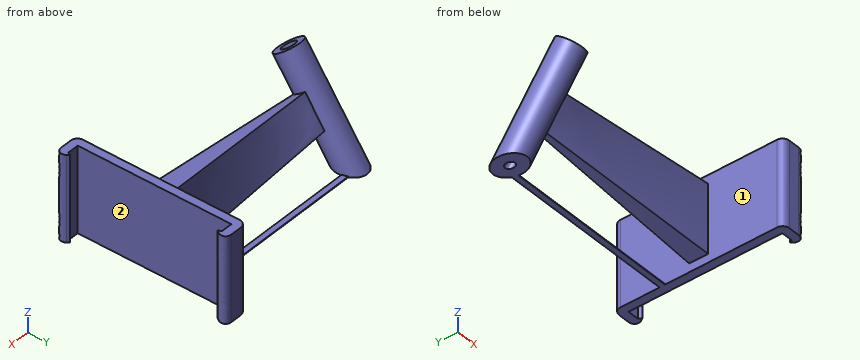
```python
from build123d import *

# Parameters (mm, degrees)
F1_DEPTH  = 25
F4_W      = 5.5
F4_H      = 20
F9_W      = 27.424
F9_H      = 9.749
F10_DEPTH = 25
F11_W     = 1.6
F11_H     = 0.2


with BuildPart() as f1:
    # F0 (on Top) → F1 (new body)
    with BuildSketch(Plane.XY):
        with BuildLine():
            Line((0, -22.4), (0, 0))
            Line((0, 0), (0, 22.4))
            Line((0, 22.4), (3.3, 22.4))
            Line((3.3, 22.4), (3.7377447908, 21.5009007295))
            Line((3.7377447908, 21.5009007295), (4.2500217799, 22.1906429157))
            add(Edge.make_bspline(
                [(4.2500217799, 22.1906429157), (4.5826178906, 22.638458401), (4.7916104177, 24.2520123151), (3.4845446819, 24.8), (2.8422182777, 24.8)],
                knots=[0, 0, 0, 0, 0.5032486408, 1, 1, 1, 1], degree=3))
            Line((2.8422182777, 24.8), (-0.4, 24.8))
            ThreePointArc((-0.4, 24.8), (-1.8142135624, 24.2142135624), (-2.4, 22.8))
            Line((-2.4, 22.8), (-2.4, 0))
            Line((-2.4, 0), (-2.4, -22.8))
            ThreePointArc((-2.4, -22.8), (-1.8142135624, -24.2142135624), (-0.4, -24.8))
            Line((-0.4, -24.8), (2.8422182777, -24.8))
            add(Edge.make_bspline(
                [(4.2500217799, -22.1906429157), (4.5826178906, -22.638458401), (4.7916104177, -24.2520123151), (3.4845446819, -24.8), (2.8422182777, -24.8)],
                knots=[0, 0, 0, 0, 0.5032486408, 1, 1, 1, 1], degree=3))
            Line((4.2500217799, -22.1906429157), (3.7377447908, -21.5009007295))
            Line((3.7377447908, -21.5009007295), (3.3, -22.4))
            Line((3.3, -22.4), (0, -22.4))
        make_face()
    extrude(amount=F1_DEPTH)

    # F4 (on face) → F5 section 0
    with BuildSketch(Plane(origin=(-2.4, 0, 0), x_dir=(0, -1, 0), z_dir=(-1, 0, 0))):
        with Locations((0, 12.5)):
            Rectangle(F4_W, F4_H)
    # F3 (on offset) → F5 section 1
    with BuildSketch(Plane.YZ.offset(-55)):
        Polygon((4.5061862703, 9.812834642), (-1.2295780932, 18.0043550849), (-4.5061862703, 15.7100493395), (1.2295780932, 7.5185288966), align=None)
    loft()

    # F7 (on face) → F8 (revolve)
    with BuildSketch(Plane(origin=(0, 5.9959164346, 4.198385886), x_dir=(1, 0, 0), z_dir=(0, -0.8191520443, -0.5735764364))):
        Polygon((-59.2, -9.0757438921), (-59.2, 15.9242561079), (-60.1, 15.9242561079), (-60.1, 25.9242561079), (-62.1, 25.9242561079), (-62.1, -9.0757438921), align=None)
    revolve(axis=Axis((-58, -0.1314634537, 12.94919126), (0, -0.5735764364, 0.8191520443)))

    # F9 (on Front) → F10 (cut)
    with BuildSketch(Plane.XZ):
        with Locations((-57.2514572268, -4.8745)):
            Rectangle(F9_W, F9_H)
    extrude(amount=-F10_DEPTH, mode=Mode.SUBTRACT)

    # F11 (on face) → F12 (join, up to the next surface of F1)
    with BuildSketch(Plane(origin=(-2.4, 0, 0), x_dir=(0, -1, 0), z_dir=(-1, 0, 0))):
        with Locations((-10.6029133692, 0.1)):
            Rectangle(F11_W, F11_H)
    extrude(until=Until.NEXT)


solid = f1.part
```
Part model, mm, in its own coordinate system. Face numbers are marked on the shaded views. Round coordinates to 2 decimals unless told otherwise and drop trailing zeros. Order: outer loops, then holes, each group sorted by start corner. A loop starts at its lowest first (then second) coordinate and runs counter-clockwise, first axis right, second up. Notation, with made-up numbers: M 19,41 L 31,41 A23 cw 31,71 Z; hole C 5,56.25 d9. An arc over 180 degrees is marked long. Put each result on its own line as item: value. Start each with the question number.
1. Slice it at A-A on z = 6.25. State how many separate pieces and enclosed holes the cut face has, then the cut area to 3 significant figures.
2. Drill centre lines: probe 1 along Z at (x, y) = (-33.5, 11); probe 2 along X at (y, z) = (12.5, 21.25); probe 3 along X at (y, z) = (22.5, 15). Where is each one in solid material? Low to high. Write a range as [from, to].
3. Drop flat-ended pins along their axis: pin 1 (2 mm diameter, centred on y = -11, z = 11, fed in from -X); pin 2 (4 mm diameter, centred on x = -49, y = 9, fed in from +Z); pin 3 (3.5 mm diameter, centred on x = 1.5, y = -5.5, fed in from +Z); pin 4 (6 mm diameter, centred on x = -36.5, y = -8, fed in from -Z). Give the stop position or say it passes through.
4. Slice it at B-B on y = 18. List the corners of the cut face in (x, z).
5. Two-plate mould, pull along Y, no slides. Class the marked faces 1 and 2: +Y half, -Y half, draft (parallel to the pull), parting line (faces both ways), or undercut.
Findings:
1. separate pieces: 2
1. enclosed holes: 1
1. area: 358 mm2
2. probe 1: [0, 0.2]
2. probe 2: [-2.4, 0]
2. probe 3: [-2.4, 4.42]
3. pin 1: x = -2.4
3. pin 2: z = 0.2
3. pin 3: z = 25
3. pin 4: through
4. outline: M -2.4,0 L 0,0 L 0,25 L -2.4,25 Z
5. face 1: draft
5. face 2: undercut
